Part model, mm, in its own coordinate system. A direction names the side the tool comes from. Round coordinates to 2 decimals unless told otherwise and drop trailing zeros. Order: outer loops, then holes, each group sorted by start corner. A loop starts at its lowest first (then second) coordinate and runs counter-clockwise, first axis right, second up. Notation, with made-up numbers: (77.5, -18.75) - (134.5, -18.75) arc R20 cw to (134.5, 9.25) - close; hole circle Ø4 at (77, -29.5). An arc over 180 degrees is marked (long way). Answer as a JSON object with one key per item and string values.
```python
from build123d import *

# Parameters (mm, degrees)
F0_R     = 24.384
F1_DEPTH = 6.35
F2_W     = 61.468
F2_H     = 6.35
F2_R     = 24.384
F3_DEPTH = 11.303
F4_R     = 2.032


with BuildPart() as f1:
    # F0 (on Top) → F1 (new body)
    with BuildSketch(Plane.XY):
        with BuildLine():
            Line((-30.734, 53.594), (-30.734, 0))
            ThreePointArc((-30.734, 0), (0, -30.734), (30.734, 0))
            Line((30.734, 0), (30.734, 53.594))
            Line((30.734, 53.594), (-30.734, 53.594))
        make_face()
        Circle(F0_R, mode=Mode.SUBTRACT)
    extrude(amount=F1_DEPTH)

    # F2 (on face) → F3 (join)
    with BuildSketch(Plane.XY.offset(6.35)):
        with Locations((0, 50.419)):
            Rectangle(F2_W, F2_H)
        with BuildLine():
            Line((30.734, 30.734), (-30.734, 30.734))
            Line((-30.734, 30.734), (-30.734, 0))
            ThreePointArc((-30.734, 0), (0, -30.734), (30.734, 0))
            Line((30.734, 0), (30.734, 30.734))
        make_face()
        Circle(F2_R, mode=Mode.SUBTRACT)
    extrude(amount=F3_DEPTH)

    # F4
    f4_edges = [f1.edges().sort_by_distance(p)[0] for p in [
        (0, -30.734, 0),
        (0, 53.594, 0),
        (30.734, 53.594, 8.8265),
        (-30.734, 53.594, 8.8265),
    ]]
    fillet(f4_edges, radius=F4_R)


solid = f1.part
```
Item 1: Tool access for faces 5 (the flat face through (0, 47.244, 12)), 6 (the flat face through (0, 50, 17.653)): list every direction of +Z, -Z, +X, -X, +Y, -Y with a clear straight run to the whole face (end or side of a thin tool).
Taken from the geometry:
{"face 5": "+Z, +X, -X", "face 6": "+Z, +X, -X, +Y, -Y"}
Item 2: Cut at D-D (y = 5). Write the cut outline in (x, z).
Taken from the geometry:
{"outline": "(-30.73, 2.03) arc R2.03 ccw to (-28.7, 0) - (-23.87, 0) - (-23.87, 17.65) - (-30.73, 17.65) - close; (23.87, 0) - (28.7, 0) arc R2.03 ccw to (30.73, 2.03) - (30.73, 17.65) - (23.87, 17.65) - close"}
Item 3: Cut at B-B (x = 0). Write the cut outline in (y, z).
Taken from the geometry:
{"outline": "(-30.73, 2.03) arc R2.03 ccw to (-28.7, 0) - (-24.38, 0) - (-24.38, 17.65) - (-30.73, 17.65) - close; (24.38, 0) - (51.56, 0) arc R2.03 ccw to (53.59, 2.03) - (53.59, 17.65) - (47.24, 17.65) - (47.24, 6.35) - (30.73, 6.35) - (30.73, 17.65) - (24.38, 17.65) - close"}
Item 4: Two-plate mould, pull along Y, no slides. Class faces 1 (the flat face through (0, 30.734, 12)), 2 (the cylindrical face through (30.155, 26.142, 0.611)), 3 (the cylindrical face through (-3.174, 24.177, 8.703)), 4 (the cylindrical face through (-30.155, 52.983, 9.733)): pulls with the +Y half, pulls with the -Y half, needs draft (parallel to the pull), parting line crosses it, or undercut.
Taken from the geometry:
{"face 1": "undercut", "face 2": "needs draft", "face 3": "undercut", "face 4": "pulls with the +Y half"}
Item 5: Cut at A-A (z = 15.75). Write the cut outline in (x, y), plus the area to 3 significant figures.
Taken from the geometry:
{"outline": "(-30.73, 0) arc R30.73 ccw to (30.73, 0) - (30.73, 30.73) - (-30.73, 30.73) - close; (-30.73, 47.24) - (30.73, 47.24) - (30.73, 51.56) arc R2.03 ccw to (28.7, 53.59) - (-28.7, 53.59) arc R2.03 ccw to (-30.73, 51.56) - close; hole circle Ø48.77 at (0, 0)", "area": "1,890 mm2"}
Item 6: Cut at C-C (z = 5.5). Write the cut outline in (x, y).
Taken from the geometry:
{"outline": "(-30.73, 0) arc R30.73 ccw to (30.73, 0) - (30.73, 51.56) arc R2.03 ccw to (28.7, 53.59) - (-28.7, 53.59) arc R2.03 ccw to (-30.73, 51.56) - close; hole circle Ø48.77 at (0, 0)"}
Item 7: Drop flat-ended pins along their axis: P1, Ø3.5, axis at x = -11.5, z = 11.5, coming from the -Y side; P2, Ø3, axis at x = -21.5, z = 8, coming from the -Y side; P3, Ø6, axis at y = -12, z = 11, coming from the +X side; P4, Ø13, axis at x = -13, y = 42.5, coming from the +Z side. Give the stop position or say it passes through.
Taken from the geometry:
{"P1": "y = -29.15", "P2": "y = -23.34", "P3": "x = 29.39", "P4": "z = 17.65"}
Item 8: Probe L1, parallel to Y at x = 0, z = 11; L2, parallel to Y at x = -8, z = 10; L3, parallel to X at y = 0.5, z = 15.75. List the from-to ranges inside material, lowest first. Write a range as from..to.
Taken from the geometry:
{"L1": "-30.73..-24.38, 24.38..30.73, 47.24..53.59", "L2": "-29.67..-23.03, 23.03..30.73, 47.24..53.59", "L3": "-30.73..-24.38, 24.38..30.73"}
